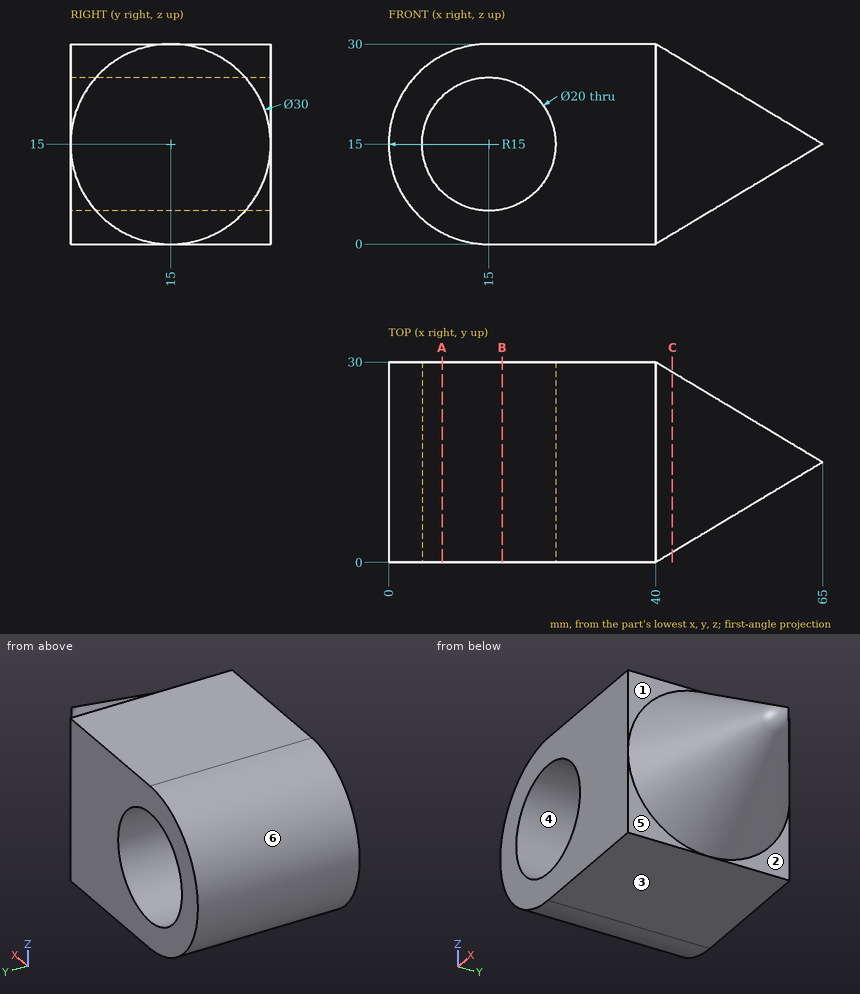
Can you work these out from the drawing? Everything is in mm from the part's minimum corner. A direction names the side the tool comes from. Give positions to 0.01 mm unless a question says otherwise; leave off trailing zeros. Order: outer loops, then holes, each group sorted by start corner. A loop starts at its lowest first (then second) coordinate and runs counter-clockwise, first axis right, second up.
Item 1: I'm going to push flat-ended pins straight in: pin 1 (4.5 mm diameter, centred on y = 24, z = 7, fed in from +X); pin 2 (12 mm diameter, centred on y = 10, z = 10.5, fed in from +X); pin 3 (2 mm diameter, centred on y = 20.5, z = 21, fed in from +X); pin 4 (1 mm diameter, centred on x = 33.5, z = 14, fed in from -Y). Where does each tip first touch, or does it pass through?
Item 2: If we mould it in two halves opening along X, with no side actions, what happens to the marked faces 4, 5 and 6? For each: pulls with the +X half, pulls with the -X half, needs draft (parallel to the pull), parting line crosses it, or undercut.
Item 3: I need wall thicknesses on line 1 (X direction, y = 1.5, z = 7); line 2 (X direction, y = 21, z = 15); line 3 (Z direction, x = 9, y = 23.75). Which ranges of each line are inside material? Lowest first, please.
Item 4: For the marked faces 1, 2 and 3, which set-ups out of +Z, -Z, +X, -X, +Y, -Y let a thin tool reach every point of the face, with its end or its side?
Item 5: If we section it at B-B, the plane x = 17: Write out the boundary of the cut face in (y, z), plus the area to 3 significant figures.
Item 6: If we section it at C-C, the plane x = 42.5: Write out the boundary of the cut face in (y, z), plus the area to 3 significant figures.
Item 7: If we section it at A-A, the plane x = 8: Write out the boundary of the cut face in (y, z), plus the area to 3 significant figures.
Values:
1. pin 1: stops at x = 48.68
1. pin 2: stops at x = 63.79
1. pin 3: stops at x = 53.1
1. pin 4: stops at y = 0
2. face 4: undercut
2. face 5: pulls with the +X half
2. face 6: pulls with the -X half
3. line 1: x = 2.31 to 9, 21 to 40
3. line 2: x = 0 to 5, 25 to 55
3. line 3: z = 1.25 to 7, 23 to 28.75
4. face 1: +Z, +X, -Y
4. face 2: -Z, +X, +Y
4. face 3: -Z, +X, -X, +Y, -Y
5. outline: (0, 0) - (30, 0) - (30, 5.2) - (0, 5.2) - close; (0, 24.8) - (30, 24.8) - (30, 30) - (0, 30) - close
5. area: 312 mm2
6. outline: circle Ø27 at (15, 15)
6. area: 573 mm2
7. outline: (0, 1.73) - (30, 1.73) - (30, 7.86) - (0, 7.86) - close; (0, 22.14) - (30, 22.14) - (30, 28.27) - (0, 28.27) - close
7. area: 368 mm2
